Model file for the job. Use its own axes, mm. Face numbers are marked on the shaded views. Round coordinates to 2 decimals unless told otherwise and drop trailing zeros. Write each loop counter-clockwise with the first axis right and the second up, starting at its lowest first coordinate (ties: lowest second). Pieces come first, ordered by that corner, then holes.
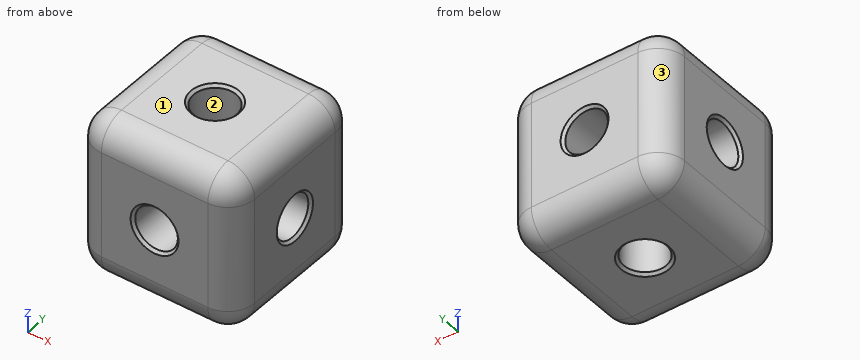
```python
from build123d import *

# Parameters (mm, degrees)
F0_W     = 30
F0_H     = 30
F1_DEPTH = 15
F2_R     = 4
F3_DEPTH = 30.001
F4_R     = 4
F5_DEPTH = 30.001
F6_R     = 4
F7_DEPTH = 30.001
F8_R     = 5
F9_SIZE  = 0.5


with BuildPart() as f1:
    # F0 (on Front) → F1 (new body, symmetric)
    with BuildSketch(Plane.XZ):
        Rectangle(F0_W, F0_H)
    extrude(amount=F1_DEPTH, both=True)

    # F2 (on face) → F3 (cut, through all)
    with BuildSketch(Plane.XZ.offset(15)):
        Circle(F2_R)
    extrude(amount=-F3_DEPTH, mode=Mode.SUBTRACT)

    # F4 (on face) → F5 (cut, through all)
    with BuildSketch(Plane.YZ.offset(15)):
        Circle(F4_R)
    extrude(amount=-F5_DEPTH, mode=Mode.SUBTRACT)

    # F6 (on face) → F7 (cut, through all)
    with BuildSketch(Plane.XY.offset(15)):
        Circle(F6_R)
    extrude(amount=-F7_DEPTH, mode=Mode.SUBTRACT)

    # F8
    f8_edges = [f1.edges().sort_by_distance(p)[0] for p in [
        (15, 0, 15),
        (0, -15, 15),
        (15, -15, 0),
        (0, -15, -15),
        (-15, -15, 0),
        (15, 15, 0),
        (0, 15, 15),
        (-15, 15, 0),
        (0, 15, -15),
        (-15, 0, 15),
        (-15, 0, -15),
        (15, 0, -15),
    ]]
    fillet(f8_edges, radius=F8_R)

    # F9
    f9_edges = [f1.edges().sort_by_distance(p)[0] for p in [
        (-4, 0, 15),
        (-4, -15, 0),
        (15, -4, 0),
        (-4, 15, 0),
        (-15, -4, 0),
        (-4, 0, -15),
    ]]
    chamfer(f9_edges, length=F9_SIZE)


solid = f1.part
```
1) Cut at A-A on y = 0. List the corners of the cut face in (x, z), and give its area (3 significant figures).
2) Wall check: probe 1 along Y at (x, z) = (9, 0); probe 2 along Z at (x, y) = (0, 10.25). Give the ranges that are in metal, low to high.
3) Flat gauge pin, fed straight in: pin 1 Ø1 at (x, y) = (-2.5, 12) entering from +Z. Where does the tip first touch, or does it go through?
4) Cut at C-C on x = -9.25. List the corners of the cut face in (y, z), and give its area (3 significant figures).
5) Pull direction X, two halves, no side cores. Call the marked faces 1, 2 and 3: released by +X, released by -X, zero draft, split by the parting line, or undercut.
Result sheet:
1. outline: (-15, -10) arc R5 ccw to (-10, -15) - (-4.5, -15) - (-4, -14.5) - (-4, -4) - (-14.5, -4) - (-15, -4.5) - close; (-15, 4.5) - (-14.5, 4) - (-4, 4) - (-4, 14.5) - (-4.5, 15) - (-10, 15) arc R5 ccw to (-15, 10) - close; (4, -14.5) - (4.5, -15) - (10, -15) arc R5 ccw to (15, -10) - (15, -4.5) - (14.5, -4) - (4, -4) - close; (4, 4) - (14.5, 4) - (15, 4.5) - (15, 10) arc R5 ccw to (10, 15) - (4.5, 15) - (4, 14.5) - close
1. area: 462 mm2
2. probe 1: y = -15 to -4, 4 to 15
2. probe 2: z = -14.99 to -4, 4 to 14.99
3. pin 1: stops at z = 14.77
4. outline: (-15, -10) arc R5 ccw to (-10, -15) - (10, -15) arc R5 ccw to (15, -10) - (15, 10) arc R5 ccw to (10, 15) - (-10, 15) arc R5 ccw to (-15, 10) - close; hole circle Ø8 at (0, 0)
4. area: 828 mm2
5. face 1: zero draft
5. face 2: undercut
5. face 3: released by -X
